Source: CAD feature listing. Evaluate the final solid. Frame: model axes, mm. A direction names the side the tool comes from. Give positions to 0.01 mm unless a question says otherwise; leave off trailing zeros. Write each loop counter-clockwise with the first axis right and the second up, starting at its lowest first coordinate (ties: lowest second). Pieces come first, ordered by that corner, then holes. Notation, with made-up numbers: (81.25, 45.5) -> (94.25, 45.5) arc R15 ccw to (94.25, 69.5) -> close; hole circle Ø4 at (42, -30.75). An arc over 180 degrees is marked (long way). Write item = value, one per line.
from build123d import *

# Parameters (mm, degrees)
SKETCH1_W           = 13.7
SKETCH1_H           = 13.7
BOSS_EXTRUDE1_DEPTH = 4
SKETCH2_R           = 6.75
BOSS_EXTRUDE2_DEPTH = 9.2
SHELL1_T            = -1


with BuildPart() as part:
    # Sketch1 → Boss-Extrude1 (new body)
    with BuildSketch(Plane(origin=(0, 0, 0), x_dir=(1, 0, 0), z_dir=(0, 1, 0))):
        Rectangle(SKETCH1_W, SKETCH1_H)
    extrude(amount=BOSS_EXTRUDE1_DEPTH)

    # Sketch2 → Boss-Extrude2 (add)
    with BuildSketch(Plane(origin=(0, 0, 0), x_dir=(1, 0, 0), z_dir=(0, 1, 0))):
        with Locations(Location((0, 0, 0), (0, 0, 90))):
            Circle(SKETCH2_R)
    extrude(amount=BOSS_EXTRUDE2_DEPTH)

    # Shell1
    shell1_openings = [part.faces().sort_by_distance(p)[0] for p in [
        (0, 9.2, 0),
        (0, 0, 0),
    ]]
    offset(amount=SHELL1_T, openings=shell1_openings, kind=Kind.INTERSECTION)


solid = part.part
1) Cut plane D-D (y = 4.5). Return the cut outline in (x, z), then the cut area to 3 significant figures.
Computed:
outline = circle Ø13.5 at (0, 0); hole circle Ø11.5 at (0, 0)
area = 39.3 mm²
2) Draft query along X for faces 4 (the flat face through (-5, 4, -5)), 5 (the flat face through (-6.85, 2, 0)), 6 (the flat face through (-5.85, 1, 0)). Return one class per face: pulls with the +X half, pulls with the -X half, needs draft (parallel to the pull), parting line crosses it, or undercut.
Computed:
face_4 = needs draft
face_5 = pulls with the -X half
face_6 = undercut
3) Cut plane B-B (x = 0). Return the cut outline in (y, z), then the cut area to 3 significant figures.
Computed:
outline = (0, -6.85) -> (4, -6.85) -> (4, -6.75) -> (9.2, -6.75) -> (9.2, -5.75) -> (3, -5.75) -> (3, -5.85) -> (0, -5.85) -> close; (0, 5.85) -> (3, 5.85) -> (3, 5.75) -> (9.2, 5.75) -> (9.2, 6.75) -> (4, 6.75) -> (4, 6.85) -> (0, 6.85) -> close
area = 18.6 mm²
4) Cut plane C-C (y = 2.5). Return the cut outline in (x, z).
Computed:
outline = (-6.85, -6.85) -> (6.85, -6.85) -> (6.85, 6.85) -> (-6.85, 6.85) -> close; hole (-5.85, -5.85) -> (5.85, -5.85) -> (5.85, 5.85) -> (-5.85, 5.85) -> close
5) Contact query for flat-ended pins moving along their axis: pin 1 (6 mm diameter, centred on x = 4, z = -2, fed in from -Y); pin 2 (1.5 mm diameter, centred on x = 4, z = -4, fed in from -Y). Output: stop coordinate, or through.
Computed:
pin_1 = 0
pin_2 = 3
6) Cut plane A-A (z = 0). Return the cut outline in (x, y), then the cut area to 3 significant figures.
Computed:
outline = (-6.85, 0) -> (-5.85, 0) -> (-5.85, 3) -> (-5.75, 3) -> (-5.75, 9.2) -> (-6.75, 9.2) -> (-6.75, 4) -> (-6.85, 4) -> close; (5.75, 3) -> (5.85, 3) -> (5.85, 0) -> (6.85, 0) -> (6.85, 4) -> (6.75, 4) -> (6.75, 9.2) -> (5.75, 9.2) -> close
area = 18.6 mm²
7) Material intervals for L1, parallel to Z at x = -1, y = 0.75; L2, parallel to X at y = 4.75, z = 0; L3, parallel to Y at x = -4, z = -5.25, sorted ascending.
Computed:
L1 = -6.85 to -5.85, 5.85 to 6.85
L2 = -6.75 to -5.75, 5.75 to 6.75
L3 = 3 to 9.2
8) Access query for faces 1 (the flat face through (-4.8, 3, -3.5)), 2 (the cylindrical face through (6.59, 6.56, 1.46)), 3 (the flat face through (0, 2, 6.85)). Directions: +Z, -Z, +X, -X, +Y, -Y. A direction counts if a zero-diameter tool reaches every point of the face in a straight line with its end or side. Return the directions, or none.
Computed:
face_1 = -Y
face_2 = +Y
face_3 = +Z, +X, -X, +Y, -Y
